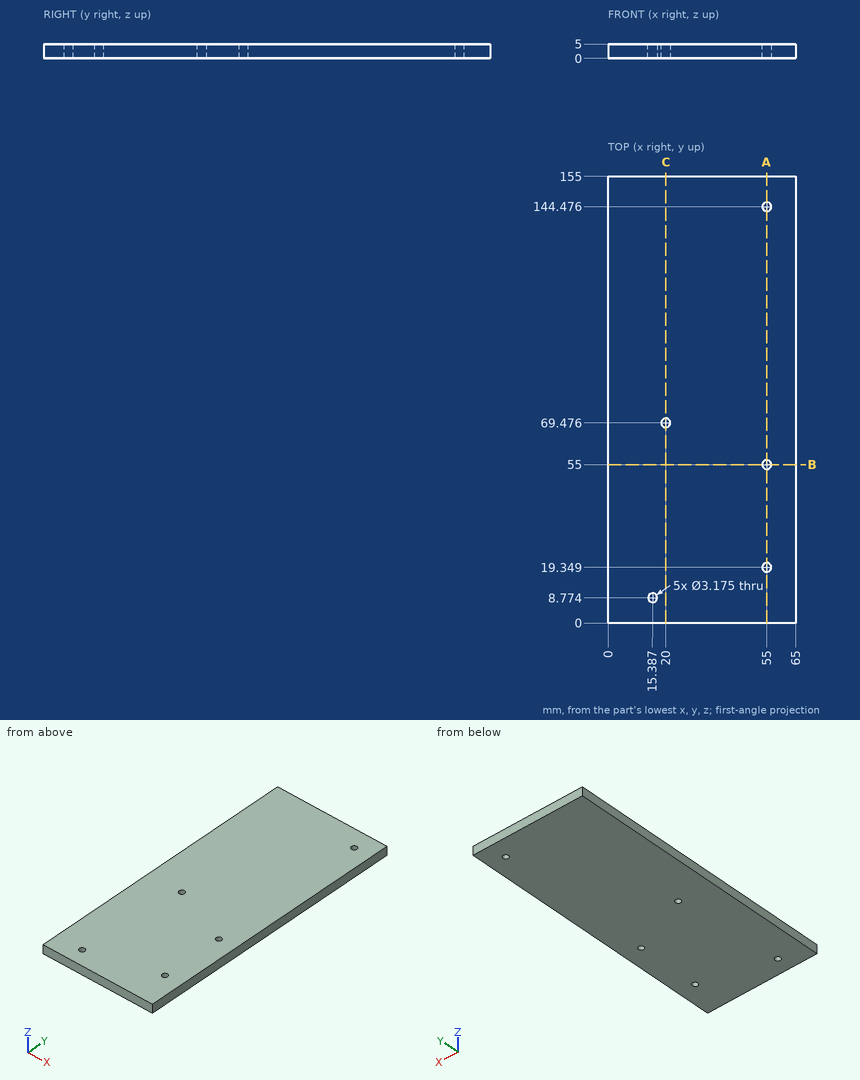
The figure shows three views and two pictorial views of one solid part (mm, origin at its lowest corner). Answer the questions. Give positions to 0.01 mm unless a question says otherwise; leave off trailing zeros. Order: outer loops, then holes, each group sorted by start corner. A loop starts at its lowest first (then second) coordinate and runs counter-clockwise, first axis right, second up. Notation, with made-up numbers: (-7.5, -20.5) -> (35.5, -20.5) arc R9 ccw to (35.5, -12.5) -> close; hole circle Ø7 at (-36.75, 60). An arc over 180 degrees is marked (long way). One line per item, written item: value.
1) Find section B-B, the plane y = 55. Determine the outline of the cut face in (x, z).
Reported:
outline: (0, 0) -> (53.41, 0) -> (53.41, 5) -> (0, 5) -> close; (56.59, 0) -> (65, 0) -> (65, 5) -> (56.59, 5) -> close
2) Find section A-A, the plane x = 55. Determine the outline of the cut face in (y, z).
Reported:
outline: (0, 0) -> (17.76, 0) -> (17.76, 5) -> (0, 5) -> close; (20.94, 0) -> (53.41, 0) -> (53.41, 5) -> (20.94, 5) -> close; (56.59, 0) -> (142.89, 0) -> (142.89, 5) -> (56.59, 5) -> close; (146.06, 0) -> (155, 0) -> (155, 5) -> (146.06, 5) -> close
3) Find section C-C, the plane x = 20. Determine the outline of the cut face in (y, z).
Reported:
outline: (0, 0) -> (67.89, 0) -> (67.89, 5) -> (0, 5) -> close; (71.06, 0) -> (155, 0) -> (155, 5) -> (71.06, 5) -> close
4) A flat-ended cylindrical pin translates along its axis: P1, Ø1.9, axis at x = 20, y = 69.48, coming from the -Z side. Find the tip coordinate at first contact, or state that the pin passes through.
Reported:
P1: passes through
5) Find the intervals of material crossed by line 1 (Y direction, x = 55, z = 1.6); line 2 (Y direction, x = 20, z = 1.95); line 3 (Y direction, x = 19, z = 4.3) (1 decimal), in increasing order.
Reported:
line 1: y = 0 to 17.76, 20.94 to 53.41, 56.59 to 142.89, 146.06 to 155
line 2: y = 0 to 67.89, 71.06 to 155
line 3: y = 0 to 68.2, 70.7 to 155
